The listing builds one solid part. Answer for the finished solid, in the listing's coordinates (mm). Face numbers are marked on the shaded views. A direction names the side the tool comes from. Round coordinates to 2 decimals unless told otherwise and drop trailing zeros. Write each loop counter-clockwise with the first axis right and the second up, starting at its lowest first coordinate (ties: lowest second). Pieces come first, ordered by that corner, then holes. Notation, with made-up numbers: M -17.75,36 L 27.25,36 A16 ccw 27.25,64 Z; hole C 49.25,70.5 d5. An arc over 180 degrees is marked long. Write each question's results on one line, items separated by ' | '.
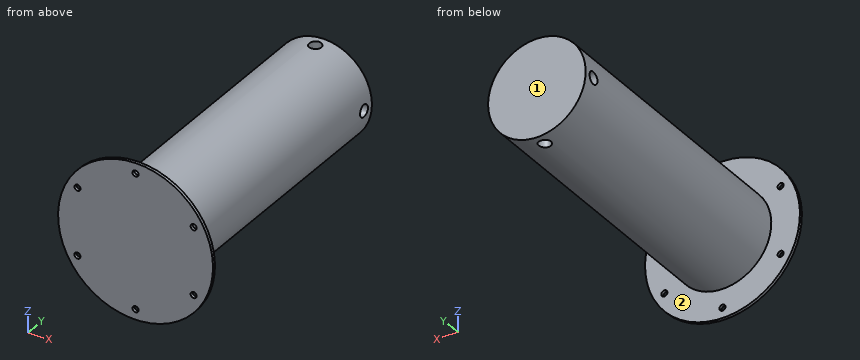
from build123d import *

# Parameters (mm, degrees)
BOSS_EXTRUDE1_START     = 8.89
SKETCH4_R               = 101.6
BOSS_EXTRUDE1_DEPTH     = 8.89
CUT_EXTRUDE2_DEPTH      = 642.371375881
CUT_EXTRUDE2_DEPTH_BACK = 642.371375881
SKETCH5_R               = 12.7
CUT_EXTRUDE3_DEPTH      = 642.371375975
CUT_EXTRUDE3_DEPTH_BACK = 642.371375975
SKETCH6_R               = 12.7
SKETCH7_R               = 6.35
CUT_EXTRUDE4_DEPTH      = 648.310167092


with BuildPart() as part:
    # Sketch2 → Revolve1 (revolve)
    with BuildSketch(Plane.XY, mode=Mode.PRIVATE) as revolve1_sk:
        Polygon((101.6, 0), (101.6, 590.55), (0, 590.55), (0, 0), (0, -6.35), (161.29, -6.35), (161.29, 0), align=None)
    revolve(revolve1_sk.sketch.rotate(Axis((0, 590.55, 0), (0, -1, 0)), 90), axis=Axis((0, 590.55, 0), (0, -1, 0)))

    # Sketch4 → Boss-Extrude1 (add)
    with BuildSketch(Plane(origin=(0, 590.55, 0), x_dir=(1, 0, 0), z_dir=(0, 1, 0)).offset(BOSS_EXTRUDE1_START)):
        with Locations(Location((0, 0, 0), (0, 0, 270))):
            Circle(SKETCH4_R)
    extrude(amount=-BOSS_EXTRUDE1_DEPTH)

    # Sketch5 → Cut-Extrude2 (cut, two sides: drawn at the far end of the back side and taken through both)
    with BuildSketch(Plane(origin=(0, 0, 0), x_dir=(0, 0, -1), z_dir=(1, 0, 0)).offset(-CUT_EXTRUDE2_DEPTH_BACK)):
        with Locations((0, 574.04)):
            Circle(SKETCH5_R)
    extrude(amount=CUT_EXTRUDE2_DEPTH + CUT_EXTRUDE2_DEPTH_BACK, mode=Mode.SUBTRACT)

    # Sketch6 → Cut-Extrude3 (cut, two sides: drawn at the far end of the back side and taken through both)
    with BuildSketch(Plane.XY.offset(-CUT_EXTRUDE3_DEPTH_BACK)):
        with Locations(Location((0, 574.04, 0), (0, 0, 270))):
            Circle(SKETCH6_R)
    extrude(amount=CUT_EXTRUDE3_DEPTH + CUT_EXTRUDE3_DEPTH_BACK, mode=Mode.SUBTRACT)

    # Sketch7 → Cut-Extrude4 (cut, through all)
    with BuildSketch(Plane.XZ.offset(6.35)):
        with Locations(Location((0, 139.7, 0), (0, 0, 270))):
            Circle(SKETCH7_R)
        with Locations(Location((120.983748909, 69.85, 0), (0, 0, 270))):
            Circle(SKETCH7_R)
        with Locations(Location((120.983748909, -69.85, 0), (0, 0, 270))):
            Circle(SKETCH7_R)
        with Locations(Location((0, -139.7, 0), (0, 0, 270))):
            Circle(SKETCH7_R)
        with Locations(Location((-120.983748909, -69.85, 0), (0, 0, 270))):
            Circle(SKETCH7_R)
        with Locations(Location((-120.983748909, 69.85, 0), (0, 0, 270))):
            Circle(SKETCH7_R)
    extrude(amount=-CUT_EXTRUDE4_DEPTH, mode=Mode.SUBTRACT)


solid = part.part
1) A tool of negligible diameter and unlimited length cuts with its end or side. For the marked faces 1 and 2, from which of +Z, -Z, +X, -X, +Y, -Y can it reach the whole face along a straight path? Write none if from no direction.
Return value:
face 1: +Z, -Z, +X, -X, +Y | face 2: +Y
2) Section B-B (z = -139.7) is taken. Determine the outline of the cut face in (x, y), then the cut area to 3 significant figures.
Return value:
outline: M -80.61,-6.35 L -6.35,-6.35 L -6.35,0 L -80.61,0 Z; M 6.35,-6.35 L 80.61,-6.35 L 80.61,0 L 6.35,0 Z | area: 943 mm²
3) Section C-C (x = 52) is taken. Determine the outline of the cut face in (y, z).
Return value:
outline: M -6.35,-152.68 L 0,-152.68 L 0,-87.28 L 599.44,-87.28 L 599.44,87.28 L 0,87.28 L 0,152.68 L -6.35,152.68 Z; hole C 574.04,0 d25.4
4) Find the intervals of material crossed by line 1 (X direction, y = -3, z = 69); line 2 (Y direction, x = 67, z = 0); line 3 (Y direction, x = 31, z = 137.5), in increasing order.
Return value:
line 1: -145.79 to -127.28, -114.69 to 114.69, 127.28 to 145.79 | line 2: -6.35 to 561.34, 586.74 to 599.44 | line 3: -6.35 to 0
5) Section A-A (z = -69.85) is taken. Determine the outline of the cut face in (x, y).
Return value:
outline: M -145.38,-6.35 L -127.33,-6.35 L -127.33,0 L -145.38,0 Z; M -114.63,-6.35 L 114.63,-6.35 L 114.63,0 L 73.78,0 L 73.78,599.44 L -73.78,599.44 L -73.78,0 L -114.63,0 Z; M 127.33,-6.35 L 145.38,-6.35 L 145.38,0 L 127.33,0 Z; hole C 0,574.04 d25.4
6) Each of these flat-tipped pins is pushed along its axis until it touches: pin 1 (20.5 mm diameter, centred on x = -120.98, z = -69.85, fed in from +Y); pin 2 (1.5 mm diameter, centred on x = -13, y = 255, fed in from -Z); pin 3 (7.5 mm diameter, centred on x = 0, z = -139.7, fed in from +Y); pin 4 (5 mm diameter, centred on y = 138.5, z = -26, fed in from +X). Where does it stop, or does it pass through?
Return value:
pin 1: y = 0 | pin 2: z = -100.86 | pin 3: through | pin 4: x = 98.84
7) Section D-D (y = 574.04) is taken. Determine the outline of the cut face in (x, z).
Return value:
outline: M -100.8,-12.7 A101.6 ccw -12.7,-100.8 L -12.7,-12.7 Z; M -100.8,12.7 L -12.7,12.7 L -12.7,100.8 A101.6 ccw Z; M 12.7,-100.8 A101.6 ccw 100.8,-12.7 L 12.7,-12.7 Z; M 12.7,12.7 L 100.8,12.7 A101.6 ccw 12.7,100.8 Z
